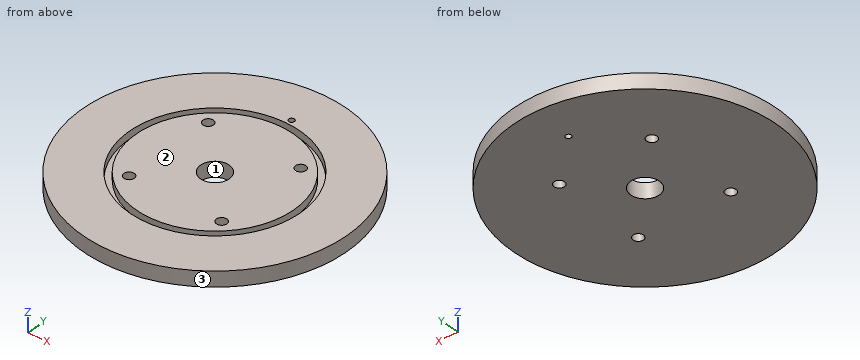
from build123d import *

# Parameters (mm, degrees)
SKETCH_1_R          = 70
SKETCH_1_R_2        = 7.6
SKETCH_1_R_3        = 2.75
SKETCH_1_R_4        = 1.5
EXTRUDE_1_DEPTH     = 8
SKETCH_2_R          = 45.2
SKETCH_2_R_2        = 41.8
CUT_EXTRUDE_2_DEPTH = 4


with BuildPart() as part:
    # 草图1 → 凸台-拉伸1 (new body)
    with BuildSketch(Plane.XY):
        Circle(SKETCH_1_R)
        Circle(SKETCH_1_R_2, mode=Mode.SUBTRACT)
        with Locations((24.748737342, 24.748737342)):
            Circle(SKETCH_1_R_3, mode=Mode.SUBTRACT)
        with Locations((-24.748737342, 24.748737342)):
            Circle(SKETCH_1_R_3, mode=Mode.SUBTRACT)
        with Locations((-24.748737342, -24.748737342)):
            Circle(SKETCH_1_R_3, mode=Mode.SUBTRACT)
        with Locations((24.748737342, -24.748737342)):
            Circle(SKETCH_1_R_3, mode=Mode.SUBTRACT)
        with Locations((0, 48)):
            Circle(SKETCH_1_R_4, mode=Mode.SUBTRACT)
    extrude(amount=-EXTRUDE_1_DEPTH)

    # 草图2 → 切除-拉伸2 (cut)
    with BuildSketch(Plane.XY):
        Circle(SKETCH_2_R)
        Circle(SKETCH_2_R_2, mode=Mode.SUBTRACT)
    extrude(amount=-CUT_EXTRUDE_2_DEPTH, mode=Mode.SUBTRACT)


solid = part.part
For this review, take the finished solid that the model builds, in its own axes (mm). Face numbers are marked on the shaded views. Give positions to 0.01 mm unless a question says otherwise; leave off trailing zeros. Loops run counter-clockwise (first coordinate to the right, second up) from the corner with the lowest first, then second, coordinate; pieces in that order, holes last.
Item 1: Take a section at B-B, the plane z = -1.75. Give the number of separate pieces and of enclosed holes in the cut face, and give its area (3 significant figures).
Item 2: Take a section at A-A, the plane y = 0. State the section outline as (x, z) points.
Item 3: Insertion check: pin 1 (7 mm diameter, centred on x = 24.75, y = -24.75, fed in from +Z); pin 2 (2 mm diameter, centred on y = -12, z = -5.5, fed in from -X); pin 3 (1.8 mm diameter, centred on x = 0, y = 48, fed in from -Z); pin 4 (1.5 mm diameter, centred on y = 54, z = -2.5, fed in from +X). Each pin has a flat end and moves straight along its axis. Give the tip position at first contact, or say it passes through.
Item 4: For line 1 along Y through (x, z) = (0, -5.75); line 2 along Y through (x, z) = (0, -3.05); line 3 along X through (y, z) = (29, -0.5), list the stretches that pass through material, from the lowest coordinate up.
Item 5: Take a section at C-C, the plane x = 17. State the section outline as (y, z) points, and give its area (3 significant figures).
Item 6: Draft analysis for pull direction Y (two halves, no side actions). For the marked faces 1, 2 and 3, state which applies: +Y half, -Y half, draft (parallel to the pull), parting line (faces both ways), or undercut.
Item 7: Take a section at D-D, the plane y = 33. State the section outline as (x, z) points.
Calculated:
1. separate pieces: 2
1. enclosed holes: 7
1. area: 14,200 mm2
2. outline: (-70, -8) - (-7.6, -8) - (-7.6, 0) - (-41.8, 0) - (-41.8, -4) - (-45.2, -4) - (-45.2, 0) - (-70, 0) - close; (7.6, -8) - (70, -8) - (70, 0) - (45.2, 0) - (45.2, -4) - (41.8, -4) - (41.8, 0) - (7.6, 0) - close
3. pin 1: stops at z = 0
3. pin 2: stops at x = -69.13
3. pin 3: passes through
3. pin 4: stops at x = 45.44
4. line 1: y = -70 to -7.6, 7.6 to 46.5, 49.5 to 70
4. line 2: y = -70 to -45.2, -41.8 to -7.6, 7.6 to 41.8, 45.2 to 46.5, 49.5 to 70
4. line 3: x = -63.71 to -34.67, -30.1 to 30.1, 34.67 to 63.71
5. outline: (-67.9, -8) - (67.9, -8) - (67.9, 0) - (41.88, 0) - (41.88, -4) - (38.19, -4) - (38.19, 0) - (-38.19, 0) - (-38.19, -4) - (-41.88, -4) - (-41.88, 0) - (-67.9, 0) - close
5. area: 1,060 mm2
6. face 1: undercut
6. face 2: draft
6. face 3: parting line
7. outline: (-61.73, -8) - (61.73, -8) - (61.73, 0) - (30.89, 0) - (30.89, -4) - (25.66, -4) - (25.66, 0) - (-25.66, 0) - (-25.66, -4) - (-30.89, -4) - (-30.89, 0) - (-61.73, 0) - close
